from build123d import *

# Parameters (mm, degrees)
F0_W       = 23
F0_H       = 14
F1_DEPTH   = 12
F2_SIZE2   = 11.99999
F2_SIZE    = 9.99999
F3_SIZE2   = 5.49999
F3_SIZE    = 11.99999
F3_2_SIZE2 = 5.49999
F3_2_SIZE  = 11.99999


# Not quite as in the source:
# - a fillet or chamfer is up to 0.001 mm smaller than in the source, because OpenCascade refuses the exact size


with BuildPart() as f1:
    # F0 (on Top) → F1 (new body)
    with BuildSketch(Plane.XY):
        Rectangle(F0_W, F0_H)
    extrude(amount=F1_DEPTH)

    # F2 (size 10 and 12 in the source; OpenCascade refuses exactly that, so slightly less here)
    f2_edges = [f1.edges().sort_by_distance(p)[0] for p in [
        (-11.5, 0, 12),
        (11.5, 0, 12),
    ]]
    f2_side = f1.faces().sort_by_distance((0, 0, 12))[0]
    chamfer(f2_edges, length=F2_SIZE, length2=F2_SIZE2, reference=f2_side)

    # F3 (size 12 and 5.5 in the source; OpenCascade refuses exactly that, so slightly less here)
    f3_edges = [f1.edges().sort_by_distance(p)[0] for p in [
        (0, -7, 12),
    ]]
    f3_side = f1.faces().sort_by_distance((0, -7, 4.461541))[0]
    chamfer(f3_edges, length=F3_SIZE, length2=F3_SIZE2, reference=f3_side)

    # F3#2 (size 12 and 5.5 in the source; OpenCascade refuses exactly that, so slightly less here)
    f3_2_edges = [f1.edges().sort_by_distance(p)[0] for p in [
        (0, 7, 12),
    ]]
    f3_2_side = f1.faces().sort_by_distance((0, 7, 4.461541))[0]
    chamfer(f3_2_edges, length=F3_2_SIZE, length2=F3_2_SIZE2, reference=f3_2_side)


solid = f1.part
Geometry check sheet. Reference: the model listing, model coordinates, mm. Coordinates: 2 decimals unless noted, no trailing zeros. Write each loop counter-clockwise with the first axis right and the second up, starting at its lowest first coordinate (ties: lowest second). Pieces come first, ordered by that corner, then holes. Notation, with made-up numbers: (-2, -30) -> (32, -30) arc R26 cw to (32, 1) -> close; hole circle Ø6 at (82, 42). An arc over 180 degrees is marked (long way). One line per question, with ' | ' between items.
1. Cross-section at C-C on z = 8.75. Record the cut outline in (x, y).
Answers:
outline: (-4.21, -2.99) -> (4.21, -2.99) -> (4.21, 2.99) -> (-4.21, 2.99) -> close
2. Cross-section at D-D on z = 2.75. Record the cut outline in (x, y), and give its area (3 significant figures).
Answers:
outline: (-9.21, -5.74) -> (9.21, -5.74) -> (9.21, 5.74) -> (-9.21, 5.74) -> close | area: 211 mm²
3. Depth check by flat-ended pin: pin 1 Ø3 at (y, z) = (3.5, 7.5) entering from +X; pin 2 Ø3 at (y, z) = (-4, 9.5) entering from +X; pin 3 Ø1 at (x, z) = (-3, 10.5) entering from -Y; pin 4 Ø2 at (x, y) = (-2.5, 3) entering from -Z. Enter the tip coordinate at first touch or a pass-through.
Answers:
pin 1: stops at x = 6.5 | pin 2: stops at x = 4.66 | pin 3: stops at y = -2.42 | pin 4: stops at z = 0
4. Thickness scan on probe 1 along Z at (x, y) = (5, -1); probe 2 along Z at (x, y) = (1, 3.5); probe 3 along Y at (x, z) = (-1, 2). Record the ranges inside material, lowest first. Write a range as from..to.
Answers:
probe 1: z = 0..7.8 | probe 2: z = 0..7.64 | probe 3: y = -6.08..6.08
